Check sheet for the drawn part. Datum: minimum x, y, z corner. Units: mm. A direction names the side the tool comes from. Coordinates: 2 decimals unless noted, no trailing zeros. Order: outer loops, then holes, each group sorted by start corner. A loop starts at its lowest first (then second) coordinate and runs counter-clockwise, first axis right, second up. Notation, with made-up numbers: M 73,21.5 L 115,21.5 A30 cw 115,53.5 Z; hole C 57.25,-28 d11. An arc over 180 degrees is marked long. Use one line per item in the form item = value. Start each with the question number.
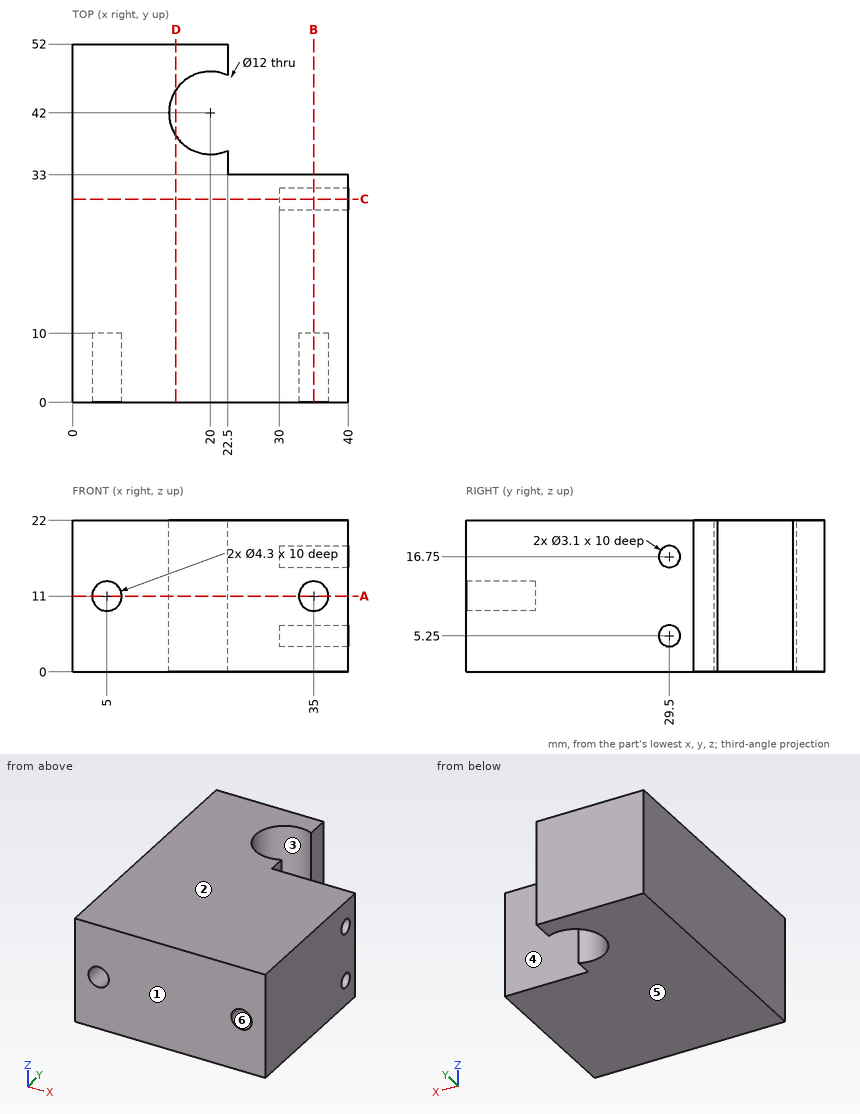
1. Cross-section at A-A on z = 11. Enter the section's corners in (x, y).
2. Cross-section at D-D on x = 15. Enter the section's corners in (y, z).
3. Material ranges on line 1 along Z through (x, y) = (35.75, 29.5); line 2 along Y through (x, z) = (20, 11.25); line 3 along Z through (x, y) = (5, 5.25), recorded low to high.
4. Cross-section at B-B on x = 35. Enter the section's corners in (y, z).
5. Depth check by flat-ended pin: P1, Ø10, axis at y = 42, z = 19.5, coming from the +X side; P2, Ø5, axis at x = 28.5, z = 7, coming from the +Y side; P3, Ø1.3, axis at x = 5, z = 10.5, coming from the -Y side; P4, Ø19, axis at x = 20, y = 42, coming from the +Z side. Enter the tip coordinate at first touch or a pass-through.
6. Cross-section at C-C on y = 29.5. Enter the section's corners in (x, z), and give its area (3 significant figures).
7. Tool access check on the marked faces 5 and 6. Record the directions out of +Z, -Z, +X, -X, +Y, -Y that give a thin tool (end or side, any length) a straight path to the whole face; none if there is none.
8. Release check for a two-part mould opening along Y. For the marked faces 1, 2, 3 and 4 record: pulls with the +Y half, pulls with the -Y half, needs draft (parallel to the pull), parting line crosses it, or undercut.
Final values:
q1.outline = M 0,0 L 2.85,0 L 2.85,10 L 7.15,10 L 7.15,0 L 32.85,0 L 32.85,10 L 37.15,10 L 37.15,0 L 40,0 L 40,33 L 22.5,33 L 22.5,36.55 A6 cw long 22.5,47.45 L 22.5,52 L 0,52 Z
q2.outline = M 0,0 L 38.68,0 L 38.68,22 L 0,22 Z; M 45.32,0 L 52,0 L 52,22 L 45.32,22 Z
q3.line_1 = 0 to 3.7, 6.8 to 15.2, 18.3 to 22
q3.line_2 = 0 to 36, 48 to 52
q3.line_3 = 0 to 8.85, 13.15 to 22
q4.outline = M 0,0 L 33,0 L 33,22 L 0,22 L 0,13.15 L 10,13.15 L 10,8.85 L 0,8.85 Z; hole C 29.5,5.25 d3.1; hole C 29.5,16.75 d3.1
q5.P1 = 16.68
q5.P2 = 33
q5.P3 = 10
q5.P4 = 22
q6.outline = M 0,0 L 40,0 L 40,3.7 L 30,3.7 L 30,6.8 L 40,6.8 L 40,15.2 L 30,15.2 L 30,18.3 L 40,18.3 L 40,22 L 0,22 Z
q6.area = 818 mm2
q7.face_5 = -Z, +X, -X, +Y, -Y
q7.face_6 = -Y
q8.face_1 = pulls with the -Y half
q8.face_2 = needs draft
q8.face_3 = undercut
q8.face_4 = pulls with the +Y half
